Read the model definition and answer for the solid it produces. Units are mm, in the model's axes. Give positions to 0.01 mm unless a question says otherwise; leave off trailing zeros. Order: outer loops, then holes, each group sorted by start corner. A loop starts at its lowest first (then second) coordinate and runs counter-clockwise, first axis right, second up. Notation, with made-up numbers: (23, 47) - (74, 47) arc R30 ccw to (74, 74) - close; hole circle Ø3 at (-15.75, 74). An arc over 180 degrees is marked (long way). One line per item, written item: value. Start each with the question number.
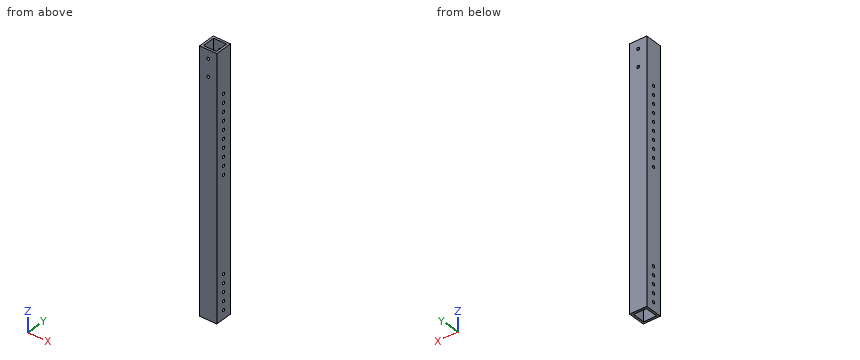
Autodesk Inventor part; units mm, degrees
ref_plane "YZ Plane" through (0, 0, 0) normal (1, 0, 0) x (0, 1, 0)
ref_plane "XZ Plane" through (0, 0, 0) normal (0, 1, 0) x (-1, 0, 0)
ref_plane "XY Plane" through (0, 0, 0) normal (0, 0, 1) x (1, 0, 0)
sketch "Sketch1" plane through (0, 0, 0) normal (0, 0, 1) x (1, 0, 0)
  line L0 (0, 0) -> (25.4, 0)
  line L1 (25.4, 0) -> (25.4, 25.4)
  line L2 (25.4, 25.4) -> (0, 25.4)
  line L3 (0, 25.4) -> (0, 0)
  line L4 (3.175, 22.225) -> (22.225, 22.225)
  line L5 (22.225, 22.225) -> (22.225, 3.175)
  line L6 (22.225, 3.175) -> (3.175, 3.175)
  line L7 (3.175, 3.175) -> (3.175, 22.225)
  dimension "d0" = 25.4
  dimension "d1" = 25.4
  dimension "d2" = 3.175
extrude "Extrusion1" add sketch "Sketch1" along normal blind 381
sketch "Sketch2" plane through (25.4, 0, 0) normal (1, 0, 0) x (0, 0, -1)
  line L0 (0, 0) -> (0, 25.4)
  line L1 (-381, 0) -> (-381, 25.4)
  line L2 (0, 0) -> (-381, 0)
  circle A0 centre (-317.5, 12.7) radius 2.0701
  circle A1 centre (-304.8, 12.7) radius 2.0701
  circle A2 centre (-292.1, 12.7) radius 2.0701
  circle A3 centre (-279.4, 12.7) radius 2.0701
  circle A4 centre (-266.7, 12.7) radius 2.0701
  circle A5 centre (-254, 12.7) radius 2.0701
  circle A6 centre (-241.3, 12.7) radius 2.0701
  circle A7 centre (-228.6, 12.7) radius 2.0701
  circle A8 centre (-215.9, 12.7) radius 2.0701
  circle A9 centre (-203.2, 12.7) radius 2.0701
  circle A10 centre (-12.7, 12.7) radius 2.0701
  circle A11 centre (-25.4, 12.7) radius 2.0701
  circle A12 centre (-38.1, 12.7) radius 2.0701
  circle A13 centre (-50.8, 12.7) radius 2.0701
  circle A14 centre (-63.5, 12.7) radius 2.0701
  dimension "d5" = 4.1402
  dimension "d6" = 12.7
  dimension "d7" = 63.5
  dimension "d10" = 12.7
  dimension "d15" = 12.7
  dimension "d16" = 12.7
  dimension "d19" = 12.7
extrude "Extrusion2" cut sketch "Sketch2" against normal blind 381
sketch "Sketch3" plane through (0, 25.4, 0) normal (0, 1, 0) x (1, 0, 0)
  line L0 (0, 0) -> (0, -381)
  line L1 (25.4, -381) -> (0, -381)
  circle A0 centre (12.7, -368.3) radius 2.0701
  circle A1 centre (12.7, -342.9) radius 2.0701
  dimension "d26" = 4.1402
  dimension "d27" = 12.7
  dimension "d28" = 12.7
  dimension "d31" = 25.4
extrude "Extrusion3" cut sketch "Sketch3" against normal blind 381
equation "\"BendRadius\" = Thickness"
equation "\"BendReliefWidth\" = Thickness"
equation "\"BendReliefDepth\" = 0.5 * Thickness"
equation "\"CornerReliefSize\" = 4 * Thickness"
equation "\"MinimumRemnant\" = 2 * Thickness"
equation "\"TransitionRadius\" = BendRadius"
equation "\"JacobiRadiusSize\" = BendRadius"
equation "\"GapSize\" = Thickness"
properties part number "Clapper 15 in Segment (4)"
1) This flat-tipped pin is pushed along its axis until it touches: pin 1 (8 mm diameter, centred on x = 8, y = 11, fed in from -Z). Where does it stop, or does it pass through?
2) Find the intervals of material crossed by probe 1 along Z at (x, y) = (12.7, 23.65); probe 2 along Y at (x, z) = (7.25, 324) (3 decimals), in increasing order. Write a range as from..to.
3) Section B-B on z = 134.5 is taken. Write down the section's boundary in (x, y) (3 decimals), plus the area to 3 significant figures.
4) Section A-A on x = 7.25 is taken. Write down the section's boundary in (y, z) (3 decimals), plus the area to 3 significant figures.
Solved:
1. pin 1: passes through
2. probe 1: z = 0..340.83, 344.97..366.23, 370.37..381
2. probe 2: y = 0..3.175, 22.225..25.4
3. outline: (0, 0) - (25.4, 0) - (25.4, 25.4) - (0, 25.4) - close; hole (3.175, 3.175) - (22.225, 3.175) - (22.225, 22.225) - (3.175, 22.225) - close
3. area: 282 mm2
4. outline: (0, 0) - (3.175, 0) - (3.175, 381) - (0, 381) - close; (22.225, 0) - (25.4, 0) - (25.4, 381) - (22.225, 381) - close
4. area: 2,420 mm2
